```python
from build123d import *

# Parameters (mm, degrees)
BOSS_EXTRUDE1_DEPTH = 40
BOSS_EXTRUDE2_DEPTH = 20
SKETCH4_R           = 5
CUT_EXTRUDE3_DEPTH  = 20


with BuildPart() as part:
    # Sketch2 → Boss-Extrude1 (new body)
    with BuildSketch(Plane.XY):
        Polygon((0, 10), (0, 0), (50, 0), (50, 18), (40, 18), (40, 8), (25, 8), (25, 18), (6.4, 18), align=None)
    extrude(amount=BOSS_EXTRUDE1_DEPTH)

    # Sketch2<4> → Boss-Extrude2 (add)
    with BuildSketch(Plane.XY):
        Polygon((20, 35), (6.4, 18), (25, 18), (25, 28), (40, 28), (40, 18), (50, 18), (50, 35), align=None)
    extrude(amount=BOSS_EXTRUDE2_DEPTH)

    # Sketch4 → Cut-Extrude3 (cut)
    with BuildSketch(Plane(origin=(0, 35, 0), x_dir=(1, 0, 0), z_dir=(0, 1, 0))):
        with Locations(Location((35, -10, 0), (0, 0, 270))):
            Circle(SKETCH4_R)
    extrude(amount=-CUT_EXTRUDE3_DEPTH, mode=Mode.SUBTRACT)


solid = part.part
```
Here's how the part is built. I have some questions about the finished solid (model axes, mm). A direction names the side the tool comes from. Coordinates: 2 decimals unless noted, no trailing zeros. Loops run counter-clockwise (first coordinate to the right, second up) from the corner with the lowest first, then second, coordinate; pieces in that order, holes last. Notation, with made-up numbers: (3.5, 53.5) - (43.5, 53.5) arc R10 cw to (43.5, 62.5) - close; hole circle Ø5 at (-33, 11). An arc over 180 degrees is marked (long way). Return JSON: item names as keys, results as strings. Group by question number.
Item 1: If we section it at A-A on x = 26.5: Write out the boundary of the cut face in (y, z).
Item 2: If we section it at B-B on y = 14: Write out the boundary of the cut face in (x, z), and give its area (3 significant figures).
Item 3: We'd pull the mould along X, two halves only. Please class faces 1 (the face through (8, 20, 15)), 2 (the face through (39, 32, 13)), 3 (the face through (40, 16, 15)), 4 (the face through (50, 13, 15)): +X half, -X half, draft (parallel to the pull), parting line (faces both ways), or undercut.
Item 4: Will these pins go through, and if not, where does the flat tip stop? P1, Ø1.5, axis at y = 19, z = 23.5, coming from the -X side; P2, Ø3, axis at y = 18, z = 19.5, coming from the -X side; P3, Ø13.5, axis at x = 33, y = 30, coming from the +Z side; P4, Ø6, axis at x = 26.5, z = 26.5, coming from the +Y side.
Item 5: If we section it at D-D on x = 35: Write out the boundary of the cut face in (y, z).
Item 6: If we section it at C-C on z = 3.5: Write out the boundary of the cut face in (x, y), and give its area (3 significant figures).
Item 7: I need wall thicknesses on line 1 (Z direction, x = 35, y = 32); line 2 (Y direction, x = 35, z = 4.5); line 3 (Y direction, x = 39, z = 35). Which ranges of each line are inside material? Lowest first, please. Write a range as from..to.
Item 8: On a 3-axis mill with a long thin cutter (end or side, diameter ignored), from which of +Z, -Z, +X, -X, +Y, -Y can I reach the whole of each face in a straight line? I mean faces 5 (the face through (29, 28, 10)), 6 (the face through (16, 18, 30)), 7 (the face through (25, 0, 20)). Say none if no direction works.
Calculated:
{
 "1": {"outline": "(0, 0) - (8, 0) - (8, 40) - (0, 40) - close; (28, 0) - (35, 0) - (35, 20) - (28, 20) - close"},
 "2": {"outline": "(3.2, 0) - (25, 0) - (25, 40) - (3.2, 40) - close; (40, 0) - (50, 0) - (50, 40) - (40, 40) - close", "area": "1,270 mm^2"},
 "3": {"face 1": "-X half", "face 2": "undercut", "face 3": "undercut", "face 4": "+X half"},
 "4": {"P1": "passes through", "P2": "stops at x = 5.2", "P3": "stops at z = 20", "P4": "stops at y = 18"},
 "5": {"outline": "(0, 0) - (8, 0) - (8, 40) - (0, 40) - close; (28, 0) - (35, 0) - (35, 5) - (28, 5) - close; (28, 15) - (35, 15) - (35, 20) - (28, 20) - close"},
 "6": {"outline": "(0, 0) - (50, 0) - (50, 35) - (20, 35) - (0, 10) - close; hole (25, 8) - (40, 8) - (40, 28) - (25, 28) - close", "area": "1,200 mm^2"},
 "7": {"line 1": "z = 0..5, 15..20", "line 2": "y = 0..8, 28..35", "line 3": "y = 0..8"},
 "8": {"face 5": "+Z, -Z", "face 6": "+Z, +X, -X, +Y", "face 7": "+Z, -Z, +X, -X, -Y"}
}
